Geometry check sheet. Reference: drawing and pictorial views, mm from the part's lowest x, y, z. A direction names the side the tool comes from. Coordinates: 2 decimals unless noted, no trailing zeros. Loops run counter-clockwise (first coordinate to the right, second up) from the corner with the lowest first, then second, coordinate; pieces in that order, holes last. Notation, with made-up numbers: M 3.25,42.25 L 27.25,42.25 A13 cw 27.25,50.25 Z; hole C 14.25,30 d5. An arc over 180 degrees is marked long. Write each question's results on one line, items separated by ' | '. Start each with the question number.
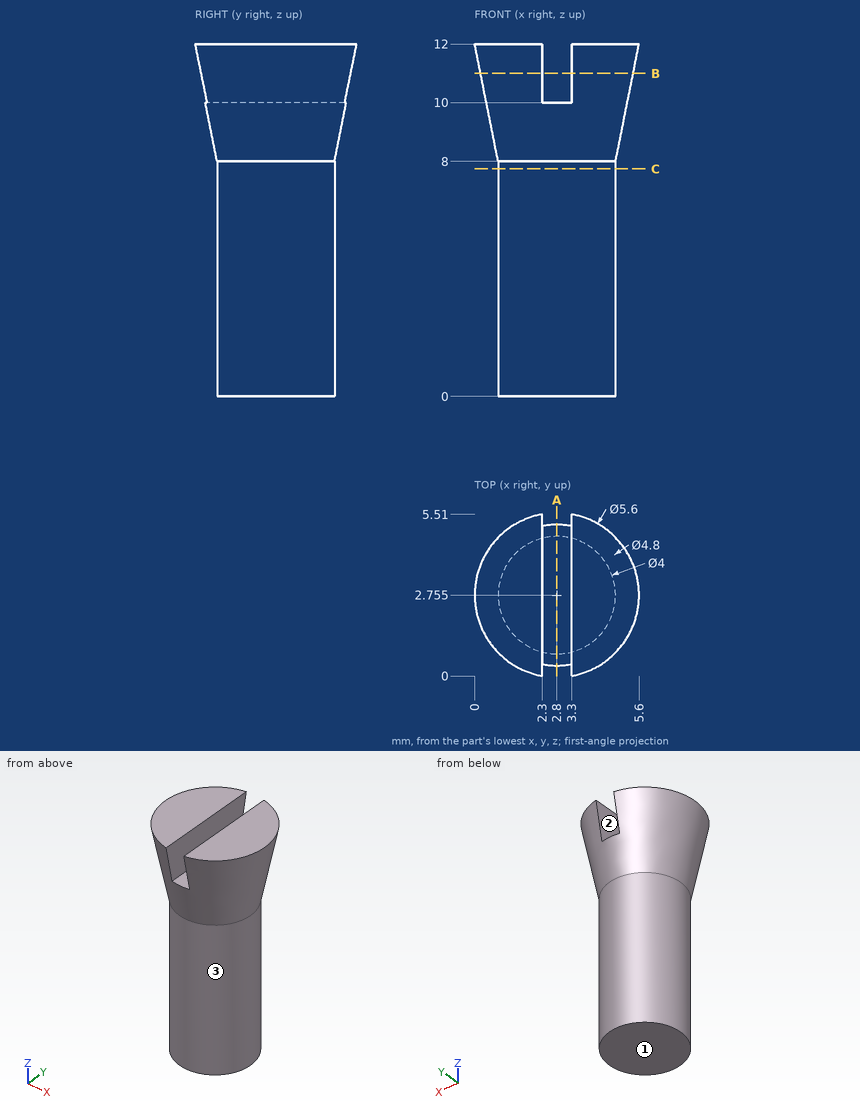
1) Gauge pin test, flat ends, axial feed: P1, Ø1.5, axis at y = 1, z = 2, coming from the -X side; P2, Ø3, axis at x = 2, z = 3, coming from the -Y side (3 decimals); P3, Ø1, axis at y = 1.5, z = 10.5, coming from the +X side. Record the tip position at first contact, or that the pin passes through.
2) Set-up check for the marked faces 1, 2 and 3: record each of +Z, -Z, +X, -X, +Y, -Y from which the full face is reachable in a straight line by a thin tool's end or side.
3) Thickness scan on probe 1 along X at (y, z) = (2.7, 7.5); probe 2 along Y at (x, z) = (2.8, 7.25) (3 decimals); probe 3 along Z at (x, y) = (3.2, 3.05). Record the ranges inside material, lowest first.
4) Section check B-B (z = 11). Enter the section's corners in (x, y) (1 decimal), then the cut area to 3 significant figures.
5) Section check A-A (x = 2.8). Enter the section's corners in (y, z) (3 decimals).
6) Section check C-C (z = 7.75). Enter the section's corners in (x, y) (3 decimals).
Return value:
1) P1: stops at x = 1.07 | P2: stops at y = 0.755 | P3: stops at x = 5.21
2) face 1: -Z, +X, -X, +Y, -Y | face 2: +Z, +Y, -Y | face 3: -Z
3) probe 1: x = 0.8 to 4.8 | probe 2: y = 0.755 to 4.755 | probe 3: z = 0 to 10
4) outline: M 2.3,0.2 L 2.3,5.3 A2.6 ccw Z; M 3.3,0.2 A2.6 ccw 3.3,5.3 Z | area: 16.1 mm2
5) outline: M 0.355,10 L 0.755,8 L 0.755,0 L 4.755,0 L 4.755,8 L 5.155,10 Z
6) outline: C 2.8,2.755 d4
